Could you check a few things on this model? Use its own coordinates, in mm. Round coordinates to 2 decimals unless told otherwise and drop trailing zeros. Write each loop counter-clockwise with the first axis right and the second up, starting at its lowest first coordinate (ties: lowest second). Pieces come first, ordered by that corner, then holes. Notation, with made-up numbers: (12, -20.5) - (57, -20.5) arc R28 cw to (57, 15.5) - close; hole circle Ø8 at (32.25, 74.5). An arc over 180 degrees is marked (long way). Put each result on its own line as item: value.
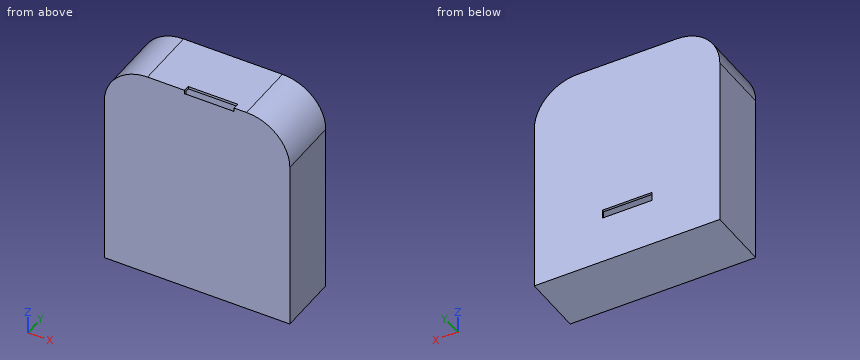
from build123d import *

# Parameters (mm, degrees)
SKETCH1_W           = 1500
SKETCH1_H           = 500
BOSS_EXTRUDE1_DEPTH = 320
SHELL1_T            = 20
SKETCH3_W           = 400
SKETCH3_H           = 70
CUT_EXTRUDE2_DEPTH  = 30
SKETCH4_W           = 1460
SKETCH4_H           = 460
CUT_EXTRUDE3_DEPTH  = 30
BOSS_EXTRUDE2_DEPTH = 500
SHELL2_START        = -230
SHELL2_DEPTH        = 460
SKETCH6_W           = 400
SKETCH6_H           = 50
CUT_EXTRUDE4_DEPTH  = 30
CHAMFER1_SIZE2      = 34.641016151
CHAMFER1_SIZE       = 20


# Read off the part's stored shape, not the designer's step: Shell2
with BuildPart() as part:
    # Sketch1 → Boss-Extrude1 (new, symmetric)
    with BuildSketch(Plane.XY):
        Rectangle(SKETCH1_W, SKETCH1_H)
    extrude(amount=BOSS_EXTRUDE1_DEPTH, both=True)

    # Shell1 (no face opened: a closed hollow body)
    add(offset(amount=-SHELL1_T, mode=Mode.PRIVATE), mode=Mode.SUBTRACT)

    # Sketch3 → Cut-Extrude2 (cut)
    with BuildSketch(Plane(origin=(0, 250, 0), x_dir=(1, 0, 0), z_dir=(0, 1, 0))):
        with Locations((0, -100)):
            Rectangle(SKETCH3_W, SKETCH3_H)
    extrude(amount=-CUT_EXTRUDE2_DEPTH, mode=Mode.SUBTRACT)

    # Sketch4 → Cut-Extrude3 (cut)
    with BuildSketch(Plane.XY.offset(320)):
        Rectangle(SKETCH4_W, SKETCH4_H)
    extrude(amount=-CUT_EXTRUDE3_DEPTH, mode=Mode.SUBTRACT)

    # Sketch5 → Boss-Extrude2 (add)
    with BuildSketch(Plane(origin=(0, 250, 0), x_dir=(1, 0, 0), z_dir=(0, 1, 0))):
        with BuildLine():
            Line((-750, -320), (750, -320))
            Line((750, -320), (750, -1070))
            ThreePointArc((750, -1070), (647.487373415, -1317.487373415), (400, -1420))
            Line((400, -1420), (-400, -1420))
            ThreePointArc((-400, -1420), (-647.487373415, -1317.487373415), (-750, -1070))
            Line((-750, -1070), (-750, -320))
        make_face()
    extrude(amount=-BOSS_EXTRUDE2_DEPTH)

    # Shell2 outline → Shell2 (cut)
    with BuildSketch(Plane(origin=(0, 0, 0), x_dir=(1, 0, 0), z_dir=(0, 1, 0)).offset(SHELL2_START)):
        with BuildLine():
            Line((730, -1070), (730, -340))
            Line((730, -340), (-730, -340))
            Line((-730, -340), (-730, -1070))
            ThreePointArc((-730, -1070), (-633.345237792, -1303.345237792), (-400, -1400))
            Line((-400, -1400), (400, -1400))
            ThreePointArc((400, -1400), (633.345237792, -1303.345237792), (730, -1070))
        make_face()
    extrude(amount=SHELL2_DEPTH, mode=Mode.SUBTRACT)

    # Sketch6 → Cut-Extrude4 (cut)
    with BuildSketch(Plane.XY.offset(1420)):
        with Locations((100, -225)):
            Rectangle(SKETCH6_W, SKETCH6_H)
    extrude(amount=-CUT_EXTRUDE4_DEPTH, mode=Mode.SUBTRACT)

    # Chamfer1
    chamfer1_edges = [part.edges().sort_by_distance(p)[0] for p in [
        (100, -230, 1390),
    ]]
    chamfer1_side = [part.faces().sort_by_distance(p)[0] for p in [
        (100, -230.4, 1390),
    ]]
    chamfer(chamfer1_edges, length=CHAMFER1_SIZE - 0.0001, length2=CHAMFER1_SIZE2 - 0.0001, reference=chamfer1_side[0])  # a hair under: the kernel refuses the full size


solid = part.part
(1) Imagine slicing it at C-C, the plane y = -148.5. List the corners of the cut face in (x, z) for me, then the cut area to 3 significant figures.
Values found:
outline: (-750, -320) - (750, -320) - (750, 1070) arc R350 ccw to (400, 1420) - (-400, 1420) arc R350 ccw to (-750, 1070) - close; hole (-730, -300) - (730, -300) - (730, 320) - (-730, 320) - close; hole (-730, 340) - (730, 340) - (730, 1070) arc R330 ccw to (400, 1400) - (-400, 1400) arc R330 ccw to (-730, 1070) - close
area: 151,000 mm^2
(2) I'm going to push a flat-ended pin straight in: pin 1 (6 mm diameter, centred on x = 148, z = 1408, fed in from -Y). Where does the tip first touch, or does it pass through?
Values found:
pin 1: stops at y = -200
(3) Imagine slicing it at A-A, the plane z = 419. List the corners of the cut face in (x, y) for me.
Values found:
outline: (-750, -250) - (750, -250) - (750, 250) - (-750, 250) - close; hole (-730, -230) - (730, -230) - (730, 230) - (-730, 230) - close
(4) Please list where these lines run through material, in increasing order: probe 1 along Z at (x, y) = (-269, 223); probe 2 along X at (y, z) = (43.5, -240); probe 3 along Y at (x, z) = (-450.5, -223). Write a range as from..to.
Values found:
probe 1: z = -320..-300, 320..340, 1400..1420
probe 2: x = -750..-730, 730..750
probe 3: y = -250..-230, 230..250
